```python
from build123d import *

# Parameters (mm, degrees)
SKETCH1_W           = 152.4
SKETCH1_H           = 152.4
BOSS_EXTRUDE1_DEPTH = 76.2
CUT_EXTRUDE1_DEPTH  = 12.7
SKETCH4_R           = 44.45
CUT_EXTRUDE2_DEPTH  = 12.7
SKETCH5_R           = 25.4
BOSS_EXTRUDE2_DEPTH = 25.4
SKETCH6_W           = 127
SKETCH6_H           = 127
CUT_EXTRUDE3_DEPTH  = 12.7


with BuildPart() as part:
    # Sketch1 → Boss-Extrude1 (new, symmetric)
    with BuildSketch(Plane(origin=(0, 0, 0), x_dir=(1, 0, 0), z_dir=(0, 1, 0))):
        Rectangle(SKETCH1_W, SKETCH1_H)
    extrude(amount=BOSS_EXTRUDE1_DEPTH, both=True)

    # Sketch2 → Cut-Revolve1 (revolve, cut)
    with BuildSketch(Plane.XY, mode=Mode.PRIVATE) as cut_revolve1_sk:
        Polygon((0, 12.7), (13.97, 12.7), (13.97, 57.15), (33.02, 76.2), (0, 76.2), align=None)
    revolve(cut_revolve1_sk.sketch.rotate(Axis((0, 0, 0), (0, 1, 0)), 90), axis=Axis((0, 0, 0), (0, 1, 0)), mode=Mode.SUBTRACT)

    # Sketch3 → Cut-Extrude1 (cut)
    with BuildSketch(Plane(origin=(76.2, 0, 0), x_dir=(0, 0, -1), z_dir=(1, 0, 0))):
        Polygon((-76.2, 44.45), (76.2, 19.05), (76.2, -19.05), (-76.2, -44.45), align=None)
    extrude(amount=-CUT_EXTRUDE1_DEPTH, mode=Mode.SUBTRACT)

    # Sketch4 → Cut-Extrude2 (cut)
    with BuildSketch(Plane.XY.offset(76.2)):
        Circle(SKETCH4_R)
    extrude(amount=-CUT_EXTRUDE2_DEPTH, mode=Mode.SUBTRACT)

    # Sketch5 → Boss-Extrude2 (add)
    with BuildSketch(Plane(origin=(0, 0, -76.2), x_dir=(-1, 0, 0), z_dir=(0, 0, -1))):
        with Locations(Location((0, 0, 0), (0, 0, 180))):
            Circle(SKETCH5_R)
    extrude(amount=BOSS_EXTRUDE2_DEPTH)

    # Sketch6 → Cut-Extrude3 (cut)
    with BuildSketch(Plane.ZY.offset(76.2)):
        Rectangle(SKETCH6_W, SKETCH6_H)
    extrude(amount=-CUT_EXTRUDE3_DEPTH, mode=Mode.SUBTRACT)


solid = part.part
```
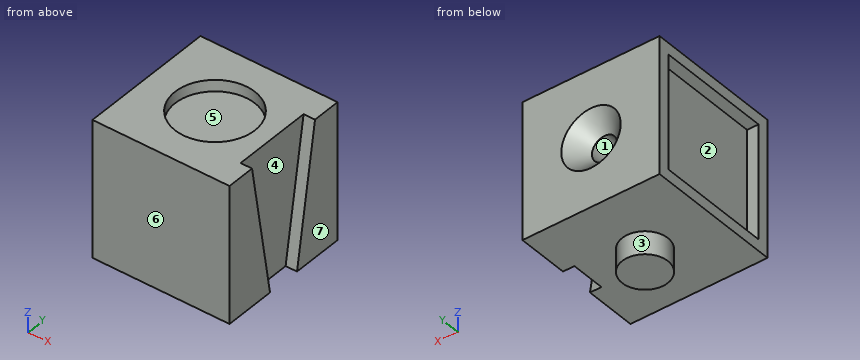
Check sheet for the modelled part. Datum: model origin and axes. Units: mm. Face numbers are marked on the shaded views. A direction names the side the tool comes from. Round coordinates to 2 decimals unless told otherwise and drop trailing zeros. Write each loop counter-clockwise with the first axis right and the second up, starting at its lowest first coordinate (ties: lowest second). Pieces come first, ordered by that corner, then holes. Notation, with made-up numbers: (-29.5, 64) -> (-23.5, 64) arc R25 ccw to (-23.5, 77) -> close; hole circle Ø7 at (1, 83). An arc over 180 degrees is marked (long way). Put each result on its own line as item: value.
(1) Sectioned sample at A-A (z = 0). Enter the section's corners in (x, y).
Values found:
outline: (-76.2, -76.2) -> (76.2, -76.2) -> (76.2, -31.75) -> (63.5, -31.75) -> (63.5, 31.75) -> (76.2, 31.75) -> (76.2, 76.2) -> (33.02, 76.2) -> (13.97, 57.15) -> (13.97, 12.7) -> (-13.97, 12.7) -> (-13.97, 57.15) -> (-33.02, 76.2) -> (-76.2, 76.2) -> (-76.2, 63.5) -> (-63.5, 63.5) -> (-63.5, -63.5) -> (-76.2, -63.5) -> close
(2) Mould release check, pull along X, two halves, no side actions. Record for the marked faces 5, 6 and 7: released by +X, released by -X, zero draft, split by the parting line, or undercut.
Values found:
face 5: undercut
face 6: zero draft
face 7: released by +X
(3) Material ranges on line 1 (Y direction, x = 0, z = 70.25); line 2 (X direction, y = 42.5, z = 0); line 3 (X direction, y = 17, z = 35), recorded low to high.
Values found:
line 1: y = -76.2 to -44.45, 44.45 to 76.2
line 2: x = -63.5 to -13.97, 13.97 to 76.2
line 3: x = -63.5 to 63.5
(4) Go/stop test with flat-tipped pins: pin 1 Ø8 at (y, z) = (3, -35) entering from +X; pin 2 Ø5 at (y, z) = (-30, 54.5) entering from -X; pin 3 Ø2 at (x, y) = (51.5, -19.5) entering from -Z. Record where each tip stops, or that it passes through.
Values found:
pin 1: stops at x = 63.5
pin 2: stops at x = -63.5
pin 3: stops at z = -76.2
(5) Tool access check on the marked faces 1, 2, 3 and 4. Record the directions out of +Z, -Z, +X, -X, +Y, -Y that give a thin tool (end or side, any length) a straight path to the whole face; none if there is none.
Values found:
face 1: +Y
face 2: -X
face 3: -Z
face 4: +Z, +X
(6) Sectioned sample at B-B (x = -66). Enter the section's corners in (y, z), plus the area to 3 significant figures.
Values found:
outline: (-76.2, -76.2) -> (76.2, -76.2) -> (76.2, 76.2) -> (-76.2, 76.2) -> close; hole (-63.5, -63.5) -> (63.5, -63.5) -> (63.5, 63.5) -> (-63.5, 63.5) -> close
area: 7,100 mm^2
(7) Sectioned sample at C-C (y = 0). Enter the section's corners in (x, z), plus the area to 3 significant figures.
Values found:
outline: (-76.2, -76.2) -> (-25.4, -76.2) -> (-25.4, -101.6) -> (25.4, -101.6) -> (25.4, -76.2) -> (63.5, -76.2) -> (63.5, 76.2) -> (44.45, 76.2) -> (44.45, 63.5) -> (-44.45, 63.5) -> (-44.45, 76.2) -> (-76.2, 76.2) -> (-76.2, 63.5) -> (-63.5, 63.5) -> (-63.5, -63.5) -> (-76.2, -63.5) -> close
area: 19,800 mm^2
(8) Sectioned sample at D-D (x = 0). Enter the section's corners in (y, z), plus the area to 4 significant figures.
Values found:
outline: (-76.2, -76.2) -> (-25.4, -76.2) -> (-25.4, -101.6) -> (25.4, -101.6) -> (25.4, -76.2) -> (76.2, -76.2) -> (76.2, -33.02) -> (57.15, -13.97) -> (12.7, -13.97) -> (12.7, 13.97) -> (57.15, 13.97) -> (76.2, 33.02) -> (76.2, 76.2) -> (44.45, 76.2) -> (44.45, 63.5) -> (-44.45, 63.5) -> (-44.45, 76.2) -> (-76.2, 76.2) -> close
area: 21,250 mm^2
